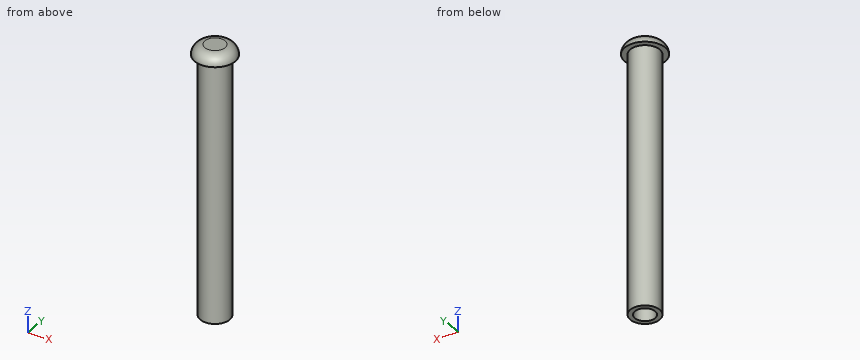
```python
from build123d import *

# Parameters (mm, degrees)
F0_R     = 3.683
F1_DEPTH = 64.77
F2_R     = 5.08
F3_DEPTH = 2.54
F4_R     = 2.53999
F5_R     = 2.54
F6_DEPTH = 12.7


# Not quite as in the source:
# - a fillet or chamfer is up to 0.001 mm smaller than in the source, because OpenCascade refuses the exact size


with BuildPart() as f1:
    # F0 (on Top) → F1 (new body)
    with BuildSketch(Plane.XY):
        Circle(F0_R)
    extrude(amount=F1_DEPTH)

    # F2 (on face) → F3 (join)
    with BuildSketch(Plane.XY.offset(64.77)):
        Circle(F2_R)
    extrude(amount=F3_DEPTH)

    # F4 (radius 2.54 in the source; OpenCascade refuses exactly that, so slightly less here)
    f4_edges = [f1.edges().sort_by_distance(p)[0] for p in [
        (-5.08, 0, 67.31),
    ]]
    fillet(f4_edges, radius=F4_R)

    # F5 (on face) → F6 (cut)
    with BuildSketch(Plane(origin=(0, 0, 0), x_dir=(1, 0, 0), z_dir=(0, 0, -1))):
        Circle(F5_R)
    extrude(amount=-F6_DEPTH, mode=Mode.SUBTRACT)


solid = f1.part
```
Read the model definition and answer for the solid it produces. Units are mm, in the model's axes. Coordinates: 2 decimals unless noted, no trailing zeros. Loops run counter-clockwise (first coordinate to the right, second up) from the corner with the lowest first, then second, coordinate; pieces in that order, holes last. Notation, with made-up numbers: (87.25, 45.5) -> (113.25, 45.5) arc R14 cw to (113.25, 64.5) -> close; hole circle Ø3 at (-6.5, 6.25). An arc over 180 degrees is marked (long way). Return JSON: item names as keys, results as strings.
Item 1: Find the intervals of material crossed by probe 1 along Y at (x, z) = (0, 6); probe 2 along Z at (x, y) = (-1, 1); probe 3 along Y at (x, z) = (0.25, 15), in increasing order.
Answers:
{"probe 1": "y = -3.68 to -2.54, 2.54 to 3.68", "probe 2": "z = 12.7 to 67.31", "probe 3": "y = -3.67 to 3.67"}
Item 2: Flat-ended cylindrical pins translate along their axes: P1, Ø1.5, axis at x = 3, z = 46, coming from the +Y side; P2, Ø1.5, axis at x = -4, z = 53.5, coming from the +Y side; P3, Ø6, axis at x = -2, z = 39, coming from the -Y side. Find the tip coordinate at first contact, or state that the pin passes through.
Answers:
{"P1": "stops at y = 2.92", "P2": "stops at y = 1.73", "P3": "stops at y = -3.68"}
Item 3: Find section C-C (z = 20.5). Determine the outline of the cut face in (x, y), plus the area to 3 significant figures.
Answers:
{"outline": "circle Ø7.37 at (0, 0)", "area": "42.6 mm2"}
